The listing builds one solid part. Answer for the finished solid, in the listing's coordinates (mm). A direction names the side the tool comes from. Coordinates: 2 decimals unless noted, no trailing zeros. Order: outer loops, then holes, each group sorted by start corner. A loop starts at its lowest first (then second) coordinate and runs counter-clockwise, first axis right, second up. Notation, with made-up numbers: (-13, -25) -> (6, -25) arc R31 ccw to (6, 14) -> close; hole circle Ø2 at (64, -24.75). An arc over 180 degrees is marked (long way). Write item = value, one per line.
from build123d import *

# Parameters (mm, degrees)
BOSS_EXTRUDE1_DEPTH = 6
CUT_EXTRUDE2_DEPTH  = 280


with BuildPart() as part:
    # Sketch1 → Boss-Extrude1 (new body)
    with BuildSketch(Plane(origin=(0, 0, 0), x_dir=(1, 0, 0), z_dir=(0, 1, 0))):
        with BuildLine():
            Line((-9.966577693, 27.987014401), (215.063422307, 27.987014401))
            ThreePointArc((215.063422307, 27.987014401), (253.954295273, 11.877887367), (270.063422307, -27.012985599))
            Line((270.063422307, -27.012985599), (270.063422307, -116.272985599))
            ThreePointArc((270.063422307, -116.272985599), (253.954295273, -155.163858564), (215.063422307, -171.272985599))
            Line((215.063422307, -171.272985599), (-9.966577693, -171.272985599))
            ThreePointArc((-9.966577693, -171.272985599), (-48.857450658, -155.163858564), (-64.966577693, -116.272985599))
            Line((-64.966577693, -116.272985599), (-64.966577693, -27.012985599))
            ThreePointArc((-64.966577693, -27.012985599), (-48.857450658, 11.877887367), (-9.966577693, 27.987014401))
        make_face()
    extrude(amount=BOSS_EXTRUDE1_DEPTH)

    # Sketch3 → Cut-Extrude2 (cut)
    with BuildSketch(Plane(origin=(0, 6, 0), x_dir=(1, 0, 0), z_dir=(0, 1, 0))):
        with BuildLine():
            Line((-10.966577693, -2.012985599), (-8.966577693, -2.012985599))
            ThreePointArc((-8.966577693, -2.012985599), (-6.845257349, -2.891665255), (-5.966577693, -5.012985599))
            Line((-5.966577693, -5.012985599), (-5.966577693, -22.417067656))
            ThreePointArc((-5.966577693, -22.417067656), (-9.966577693, -62.012985599), (-13.966577693, -22.417067656))
            Line((-13.966577693, -22.417067656), (-13.966577693, -5.012985599))
            ThreePointArc((-13.966577693, -5.012985599), (-13.087898036, -2.891665255), (-10.966577693, -2.012985599))
        make_face()
        with BuildLine():
            Line((214.063422307, -2.012985599), (216.063422307, -2.012985599))
            ThreePointArc((216.063422307, -2.012985599), (218.184742651, -2.891665255), (219.063422307, -5.012985599))
            Line((219.063422307, -5.012985599), (219.063422307, -22.417067656))
            ThreePointArc((219.063422307, -22.417067656), (215.063422307, -62.012985599), (211.063422307, -22.417067656))
            Line((211.063422307, -22.417067656), (211.063422307, -5.012985599))
            ThreePointArc((211.063422307, -5.012985599), (211.942101964, -2.891665255), (214.063422307, -2.012985599))
        make_face()
    extrude(amount=-CUT_EXTRUDE2_DEPTH, mode=Mode.SUBTRACT)


solid = part.part
Q1. Find the intervals of material crossed by line 1 along X through (y, z) = (3.6, 31); line 2 along Z through (x, y) = (-10.5, 4.2); line 3 along Z through (x, y) = (3, 5.6), in increasing order.
The answers:
line_1 = -64.97 to -26.66, 6.73 to 198.37, 231.76 to 270.06
line_2 = -27.98 to 2.01, 62.01 to 171.27
line_3 = -27.99 to 26.79, 57.24 to 171.27
Q2. A tool of negligible diameter and unlimited length cuts with its end or side. For faces 1 (the face through (-49.28, 2.96, -11.45)), 2 (the face through (219.063, 3, 14)), from which of +Z, -Z, +X, -X, +Y, -Y can it reach the whole face along a straight path? Write none if from no direction.
The answers:
face_1 = -Z, -X, +Y, -Y
face_2 = +Y, -Y
Q3. Section B-B, the plane x = 206 is taken. Give the vertices of the cut face in (y, z).
The answers:
outline = (0, -27.99) -> (6, -27.99) -> (6, 24.18) -> (0, 24.18) -> close; (0, 59.84) -> (6, 59.84) -> (6, 171.27) -> (0, 171.27) -> close
Q4. Section A-A, the plane y = 1.6 is taken. Give the vertices of the cut face in (x, z), plus the area to 3 significant figures.
The answers:
outline = (-64.97, 27.01) arc R55 ccw to (-9.97, -27.99) -> (215.06, -27.99) arc R55 ccw to (270.06, 27.01) -> (270.06, 116.27) arc R55 ccw to (215.06, 171.27) -> (-9.97, 171.27) arc R55 ccw to (-64.97, 116.27) -> close; hole (-13.97, 5.01) arc R3 ccw to (-10.97, 2.01) -> (-8.97, 2.01) arc R3 ccw to (-5.97, 5.01) -> (-5.97, 22.42) arc R20 ccw (long way) to (-13.97, 22.42) -> close; hole (211.06, 5.01) arc R3 ccw to (214.06, 2.01) -> (216.06, 2.01) arc R3 ccw to (219.06, 5.01) -> (219.06, 22.42) arc R20 ccw (long way) to (211.06, 22.42) -> close
area = 61,300 mm2
Q5. Section C-C, the plane z = 57.5 is taken. Give the vertices of the cut face in (x, y).
The answers:
outline = (-64.97, 0) -> (-22.62, 0) -> (-22.62, 6) -> (-64.97, 6) -> close; (2.69, 0) -> (202.41, 0) -> (202.41, 6) -> (2.69, 6) -> close; (227.72, 0) -> (270.06, 0) -> (270.06, 6) -> (227.72, 6) -> close
Q6. Each of these flat-tipped pins is pushed along its axis until it touches: pin 1 Ø2 at (x, y) = (215.5, 2.5) entering from +Z; pin 2 Ø1.8 at (y, z) = (3, 13) entering from +X; pin 3 Ø3 at (y, z) = (4.5, 15) entering from -X. Where does it stop, or does it pass through?
The answers:
pin_1 = 171.27
pin_2 = 268.48
pin_3 = -63.95
Q7. Section D-D, the plane x = -24.5 is taken. Give the vertices of the cut face in (y, z).
The answers:
outline = (0, -26.03) -> (6, -26.03) -> (6, 28.27) -> (0, 28.27) -> close; (0, 55.75) -> (6, 55.75) -> (6, 169.32) -> (0, 169.32) -> close
